```python
from build123d import *

# Parameters (mm, degrees)
SKETCH3_R          = 2.098913331
CUT_EXTRUDE1_DEPTH = 60


# Read off the part's stored shape, not the designer's step: #12-24 Machine Threads Stud1
with BuildPart() as part:
    # Sketch2 → Revolve1 (revolve)
    with BuildSketch(Plane.XY, mode=Mode.PRIVATE) as revolve1_sk:
        Polygon((0, 0), (0, 25), (-3.15, 25), (-3.15, 17), (-5, 17), (-5, 13), (-2.65, 13), (-2.65, 0), align=None)
    revolve(revolve1_sk.sketch.rotate(Axis((0, 0, 0), (0, 1, 0)), 270), axis=Axis((0, 0, 0), (0, 1, 0)))

    # Sketch3 → Cut-Extrude1 (cut)
    with BuildSketch(Plane(origin=(0, 25, 0), x_dir=(1, 0, 0), z_dir=(0, 1, 0))):
        with Locations(Location((0, 0, 0), (0, 0, 270))):
            Circle(SKETCH3_R)
    extrude(amount=-CUT_EXTRUDE1_DEPTH, mode=Mode.SUBTRACT)

    # #12-24 Machine Threads Stud1 outline → #12-24 Machine Threads Stud1 (revolve, cut)
    with BuildSketch(Plane.XY):
        Polygon((2.7432, 24.37008), (2.7432, 17), (3.15, 17), (3.15, 25), (2.11328, 25), align=None)
    revolve(axis=Axis((0, 0, 0), (0, 1, 0)), mode=Mode.SUBTRACT)


solid = part.part
```
Here's how the part is built. I have some questions about the finished solid (model axes, mm). A direction names the side the tool comes from. Give positions to 0.01 mm unless a question says otherwise; leave off trailing zeros. Order: outer loops, then holes, each group sorted by start corner. A loop starts at its lowest first (then second) coordinate and runs counter-clockwise, first axis right, second up. Notation, with made-up numbers: M 50.25,1 L 90.25,1 A32 ccw 90.25,37 Z; hole C 80,-17 d4. An arc over 180 degrees is marked long. Use a Markdown table: item, result. Add a question column.
1. I need wall thicknesses on probe 1 along X at (y, z) = (18, 0); probe 2 along X at (y, z) = (9, 0); probe 3 along Y at (x, z) = (3.75, 0). Which ranges of each line are inside material? Lowest first, please. Write a range as from..to.
2. On a 3-axis mill with a long thin cutter (end or side, diameter ignored), from which of +Z, -Z, +X, -X, +Y, -Y can I reach the whole of each face in a straight line? I mean faces 1 (the flat face through (-2.2, 17, 2.2)), 2 (the cylindrical face through (4.88, 14.97, 1.08)). Say none if no direction works.
3. If we mould it in two halves opening along Z, with no side actions, what happens to faces 3 (the cylindrical face through (1.419, 12.675, -1.547)), 4 (the cylindrical face through (1.612, 6.409, 2.103)), 5 (the flat face through (2, 13, -2))? For each: +Z half, -Z half, draft (parallel to the pull), parting line (faces both ways), or undercut.
4. Suppose I cut it at C-C (y = 20.5). List the corners of the cut face in (x, z) for me, and give its area (3 significant figures).
5. Suppose I cut it at D-D (x = 4). List the corners of the cut face in (y, z) for me, and give its area (3 significant figures).
6. For pin 1 Ø1 at (x, z) = (-2, -2.5) entering from +Y; pin 2 Ø6 at (y, z) = (18, -1.5) entering from -X; pin 3 Ø4 at (x, z) = (0, 0) entering from +Y; pin 4 Ø5 at (x, y) = (3, 4.5) entering from +Z, each with a flat end and sliding along its axis, tell me the tip position at first contact or that it passes through.
Results list:
| question | item | result |
|---|---|---|
| 1 | probe 1 | x = -2.74..-2.1, 2.1..2.74 |
| 1 | probe 2 | x = -2.65..-2.1, 2.1..2.65 |
| 1 | probe 3 | y = 13..17 |
| 2 | face 1 | +Y |
| 2 | face 2 | +Y, -Y |
| 3 | face 3 | undercut |
| 3 | face 4 | parting line |
| 3 | face 5 | draft |
| 4 | outline | C 0,0 d5.49; hole C 0,0 d4.2 |
| 4 | area | 9.80 mm² |
| 5 | outline | M 13,-3 L 17,-3 L 17,3 L 13,3 Z |
| 5 | area | 24.0 mm² |
| 6 | pin 1 | stops at y = 24.41 |
| 6 | pin 2 | stops at x = -5 |
| 6 | pin 3 | passes through |
| 6 | pin 4 | stops at z = 2.6 |
